```python
from build123d import *

# Parameters (mm, degrees)
F0_W     = 7
F0_H     = 11
F2_R     = 22
F2_R_2   = 16
F3_DEPTH = 25
F4_R     = 11.5
F5_DEPTH = 25


with BuildPart() as f1:
    # F0 (on Top) → F1 (revolve)
    with BuildSketch(Plane.XY):
        with Locations((3.5, 5.5)):
            Rectangle(F0_W, F0_H)
        with BuildLine():
            Line((0, 16), (0, 11))
            Line((0, 11), (7, 11))
            Line((7, 11), (7, 16))
            ThreePointArc((7, 16), (3.5, 12.5), (0, 16))
        make_face()
    revolve(axis=Axis((3.5, 0, 0), (1, 0, 0)))

    # F2 (on face) → F3 (cut)
    with BuildSketch(Plane(origin=(0, 0, 0), x_dir=(0, -1, 0), z_dir=(-1, 0, 0))):
        Circle(F2_R)
        Circle(F2_R_2, mode=Mode.SUBTRACT)
    extrude(amount=-F3_DEPTH, mode=Mode.SUBTRACT)

    # F4 (on face) → F5 (cut)
    with BuildSketch(Plane(origin=(0, 0, 0), x_dir=(0, -1, 0), z_dir=(-1, 0, 0))):
        Circle(F4_R)
    extrude(amount=-F5_DEPTH, mode=Mode.SUBTRACT)


solid = f1.part
```
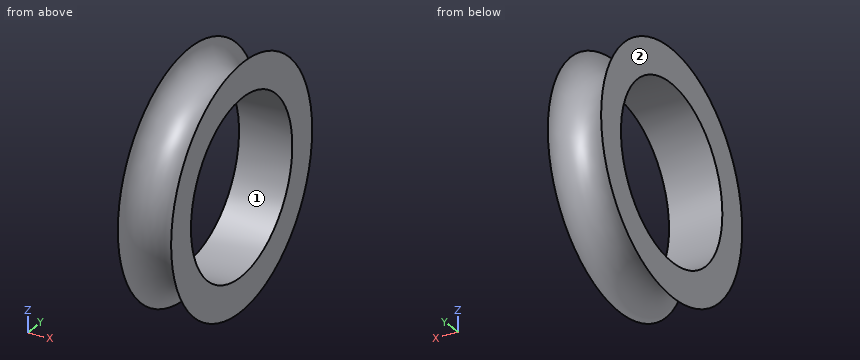
CAD build for the part. Positions are in the model's coordinates, mm. Face numbers are marked on the shaded views. Coordinates: 2 decimals unless noted, no trailing zeros. Order: outer loops, then holes, each group sorted by start corner. A loop starts at its lowest first (then second) coordinate and runs counter-clockwise, first axis right, second up.
(1) Saw through at C-C, the plane x = 0.5. Write the cut outline in (y, z).
Solution:
outline: circle Ø28.39 at (0, 0); hole circle Ø23 at (0, 0)
(2) Pin check, flat tips, straight feed: pin 1 Ø4 at (x, y) = (3.5, 11.5) entering from -Z; pin 2 Ø1 at (x, y) = (5.5, -9) entering from -Z. Stop position of each tip, or through.
Solution:
pin 1: stops at z = -8.12
pin 2: stops at z = -10.26
(3) Drill centre lines: L1, parallel to Z at x = 2, y = 0; L2, parallel to Y at x = 4.75, z = -10; L3, parallel to Y at x = 5.5, z = 9. Where is each one in solid material? Low to high.
Solution:
L1: z = -12.84 to -11.5, 11.5 to 12.84
L2: y = -7.88 to -5.68, 5.68 to 7.88
L3: y = -9.56 to -7.16, 7.16 to 9.56
(4) Saw through at D-D, the plane x = 6. Write the cut outline in (y, z), and give its area (3 significant figures).
Solution:
outline: circle Ø27.1 at (0, 0); hole circle Ø23 at (0, 0)
area: 161 mm2
(5) Mould opens along Y. For the marked faces 1 and 2 say: released by +Y, released by -Y, zero draft, split by the parting line, or undercut.
Solution:
face 1: undercut
face 2: zero draft
(6) Saw through at A-A, the plane y = 0. Write the cut outline in (x, z).
Solution:
outline: (0, -16) arc R3.5 cw to (7, -16) - (7, -11.5) - (0, -11.5) - close; (0, 11.5) - (7, 11.5) - (7, 16) arc R3.5 cw to (0, 16) - close
